Input: dimensioned drawing with shaded views. Units: mm. Origin: part minimum x, y, z. A direction names the side the tool comes from. Coordinates: 2 decimals unless noted, no trailing zeros. Loops run counter-clockwise (first coordinate to the right, second up) from the corner with the lowest first, then second, coordinate; pieces in that order, holes last. Notation, with made-up numbers: (-16, -7) -> (20, -7) arc R17 cw to (20, 13) -> close; hole circle Ø9 at (77.25, 66). An arc over 180 degrees is marked (long way). Answer as CSV lines item,"result".
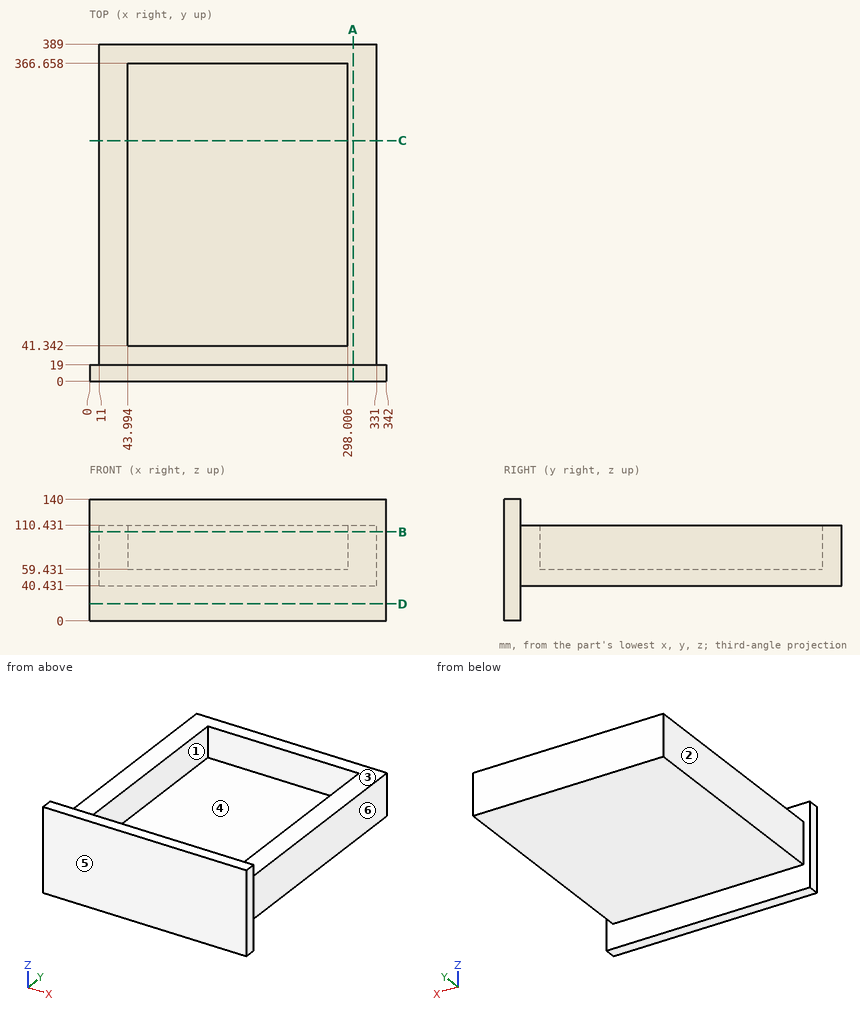
(1) Material intervals for L1, parallel to Y at x = 248.5, z = 64; L2, parallel to Y at x = 210, z = 113.5; L3, parallel to Z at x = 176, y = 164, sorted ascending. Write a range as [from, to].
Computed values:
L1,"[0, 41.34], [366.66, 389]"
L2,"[0, 19]"
L3,"[40.43, 59.43]"
(2) Cut plane C-C (y = 277.5). Return the cut outline in (x, z).
Computed values:
outline,"(11, 40.43) -> (331, 40.43) -> (331, 110.43) -> (298.01, 110.43) -> (298.01, 59.43) -> (43.99, 59.43) -> (43.99, 110.43) -> (11, 110.43) -> close"
(3) Access query for the marked faces 1, 2 and 3. Directions: +Z, -Z, +X, -X, +Y, -Y. A direction counts if a zero-diameter tool reaches every point of the face in a straight line with its end or side. Return the directions, or none.
Computed values:
face 1,"+Z"
face 2,"+Z, -Z, -X, +Y"
face 3,"+Z, +X, -X, +Y"
(4) Cut plane B-B (z = 102.5). Return the cut outline in (x, y), then the cut area to 3 significant figures.
Computed values:
outline,"(0, 0) -> (342, 0) -> (342, 19) -> (331, 19) -> (331, 389) -> (11, 389) -> (11, 19) -> (0, 19) -> close; hole (43.99, 41.34) -> (298.01, 41.34) -> (298.01, 366.66) -> (43.99, 366.66) -> close"
area,"42,300 mm^2"
(5) Pin query (flat end, axial travel): pin 1 Ø4 at (y, z) = (301.5, 98.5) entering from +X; pin 2 Ø10 at (x, y) = (172, 67) entering from -Z; pin 3 Ø2 at (x, y) = (292, 294) entering from +Z. Return the tip coordinate at first contact, or that it passes through.
Computed values:
pin 1,"x = 331"
pin 2,"z = 40.43"
pin 3,"z = 59.43"
(6) Cut plane A-A (x = 304). Return the cut outline in (y, z).
Computed values:
outline,"(0, 0) -> (19, 0) -> (19, 40.43) -> (389, 40.43) -> (389, 110.43) -> (19, 110.43) -> (19, 140) -> (0, 140) -> close"
(7) Cut plane D-D (z = 19.5). Return the cut outline in (x, y).
Computed values:
outline,"(0, 0) -> (342, 0) -> (342, 19) -> (0, 19) -> close"
(8) Draft query along Y for the marked faces 4, 5 and 6. Return one class per face: released by +Y, released by -Y, zero draft, split by the parting line, or undercut.
Computed values:
face 4,"undercut"
face 5,"released by -Y"
face 6,"zero draft"
